Input: part model. Units: mm. Frame: model coordinates. A direction names the side the tool comes from. Round coordinates to 2 decimals unless told otherwise and drop trailing zeros. Loops run counter-clockwise (first coordinate to the right, second up) from the corner with the lowest first, then second, coordinate; pieces in that order, holes last. Notation, with made-up numbers: M 50.5,39 L 93.5,39 A8 ccw 93.5,53 Z; hole C 86.5,-24.75 d11. An arc over 180 degrees is marked long. Return JSON: item names as keys, results as strings. Group by question number.
1) Section C-C (z = 9.5). Output: boundary loops of the cut face in (x, y), plus the area to 3 significant figures.
2) Section B-B (y = 9). Output: boundary loops of the cut face in (x, z).
3) Section A-A (x = -106). Output: boundary loops of the cut face in (y, z).
4) Access query for faces 1 (the face through (-91, 15, 50)), 2 (the face through (-89.792, 5, 15)), 3 (the face through (-89.722, 30, 40)), 4 (the face through (-100, 14.985, 15)). Directions: +Z, -Z, +X, -X, +Y, -Y. A direction counts if a zero-diameter tool reaches every point of the face in a straight line with its end or side. Return the directions, or none.
5) Section D-D (y = 30). Output: boundary loops of the cut face in (x, z), plus the area to 3 significant figures.
6) Contact query for flat-ended pins moving along their axis: P1, Ø22, axis at x = -101.5, z = 17, coming from the +Y side; P2, Ø10, axis at y = 4.5, z = 19.5, coming from the +X side; P3, Ø6, axis at y = 22.5, z = 38.5, coming from the +X side. Output: stop coordinate, or through.
7) Material intervals for line 1 (X direction, y = 12, z = 23.5); line 2 (Z direction, x = -103, y = 22); line 3 (Y direction, x = -91.5, z = 14.5), sorted ascending. Write a range as from..to.
from build123d import *

# Parameters (mm, degrees)
ESQUISSE2_W                  = 50
ESQUISSE2_H                  = 50
BOSS_EXTRU_1_DEPTH           = 50
ENL_V_MAT_EXTRU_1_DEPTH      = 129.695677467
ENL_V_MAT_EXTRU_1_DEPTH_BACK = 50
ENL_V_MAT_EXTRU_2_DEPTH      = 129.695677467
ENL_V_MAT_EXTRU_2_DEPTH_BACK = 30
ENL_V_MAT_EXTRU_3_DEPTH      = 129.695677467
ENL_V_MAT_EXTRU_3_DEPTH_BACK = 30


with BuildPart() as part:
    # Esquisse2 → Boss.-Extru.1 (new body)
    with BuildSketch(Plane.XY):
        with Locations((-84.722222222, 19.984567901)):
            Rectangle(ESQUISSE2_W, ESQUISSE2_H)
    extrude(amount=BOSS_EXTRU_1_DEPTH)

    # Esquisse3 → Enlèv. mat.-Extru.1 (cut, two sides: drawn at the far end of the back side and taken through both)
    with BuildSketch(Plane.XY.offset(50).offset(-ENL_V_MAT_EXTRU_1_DEPTH_BACK)):
        Polygon((-89.722222222, 171.603605798), (-89.722222222, 44.984567901), (-89.722222222, 14.984567901), (-59.722222222, 14.984567901), (66.896815675, 14.984567901), (245.963176323, 194.05092855), (89.344138426, 350.669966447), align=None)
    extrude(amount=ENL_V_MAT_EXTRU_1_DEPTH + ENL_V_MAT_EXTRU_1_DEPTH_BACK, mode=Mode.SUBTRACT)

    # Esquisse4 → Enlèv. mat.-Extru.2 (cut, two sides: drawn at the far end of the back side and taken through both)
    with BuildSketch(Plane(origin=(0, 0, 0), x_dir=(-1, 0, 0), z_dir=(0, 0, -1)).offset(-ENL_V_MAT_EXTRU_2_DEPTH_BACK)):
        Polygon((-36.896815675, 14.984567901), (89.722222222, 14.984567901), (109.722222222, 14.984567901), (236.341260119, 14.984567901), (236.341260119, 268.222643695), (-36.896815675, 268.222643695), align=None)
    extrude(amount=ENL_V_MAT_EXTRU_2_DEPTH + ENL_V_MAT_EXTRU_2_DEPTH_BACK, mode=Mode.SUBTRACT)

    # Esquisse5 → Enlèv. mat.-Extru.3 (cut, two sides: drawn at the far end of the back side and taken through both)
    with BuildSketch(Plane(origin=(0, 0, 0), x_dir=(-1, 0, 0), z_dir=(0, 0, -1)).offset(-ENL_V_MAT_EXTRU_3_DEPTH_BACK)):
        Polygon((89.792498294, 141.675981519), (89.792498294, 14.984567901), (89.792498294, -5.015432099), (89.792498294, -131.706845716), (-163.590328941, -131.706845716), (-163.590328941, 141.675981519), align=None)
    extrude(amount=ENL_V_MAT_EXTRU_3_DEPTH + ENL_V_MAT_EXTRU_3_DEPTH_BACK, mode=Mode.SUBTRACT)


solid = part.part
Returned:
{
 "1": {"outline": "M -109.72,-5.02 L -89.79,-5.02 L -89.79,14.98 L -109.72,14.98 Z", "area": "399 mm^2"},
 "2": {"outline": "M -109.72,0 L -89.79,0 L -89.79,30 L -59.72,30 L -59.72,50 L -109.72,50 Z"},
 "3": {"outline": "M -5.02,0 L 14.98,0 L 14.98,30 L 44.98,30 L 44.98,50 L -5.02,50 Z"},
 "4": {"face 1": "+Z, +X, -X, +Y, -Y", "face 2": "-Z, +X, +Y, -Y", "face 3": "+Z, -Z, +X, +Y", "face 4": "-Z, +X, -X, +Y"},
 "5": {"outline": "M -109.72,30 L -89.72,30 L -89.72,50 L -109.72,50 Z", "area": "400 mm^2"},
 "6": {"P1": "stops at y = 14.98", "P2": "stops at x = -89.79", "P3": "stops at x = -89.72"},
 "7": {"line 1": "x = -109.72..-89.79", "line 2": "z = 30..50", "line 3": "y = -5.02..14.98"}
}
